Design review of the part built by this model. Coordinates are the model's own, in mm. A direction names the side the tool comes from. Round coordinates to 2 decimals unless told otherwise and drop trailing zeros. Loops run counter-clockwise (first coordinate to the right, second up) from the corner with the lowest first, then second, coordinate; pieces in that order, holes last. Notation, with made-up numbers: (68.5, 68) - (89.5, 68) arc R15 ccw to (89.5, 80) - close; hole circle Ø5 at (0.5, 21). An arc over 180 degrees is marked (long way). Return JSON: item names as keys, results as strings. Group by question number.
(1) We need section A-A, the plane x = 30. Write out the cut boundary in (y, z), and give its area (3 significant figures).
(2) The part is to be moulded in two halves that separate along Y. For faces 4 (the cylindrical face through (1, 2, 2)), 5 (the flat face through (44, 48, 4)), 6 (the flat face through (0, 65, 3)), say which applies: pulls with the +Y half, pulls with the -Y half, needs draft (parallel to the pull), parting line crosses it, or undercut.
(3) We need section B-B, the plane z = 41.5. Give the number of separate pieces and of enclosed holes in the cut face, and give its area (4 significant figures).
(4) For faces 1 (the flat face through (24, 24, 51)), 2 (the flat face through (1.5, 92, 25)), 3 (the flat face through (3, 92, 25)), list the 3-axis set-ups (+Z, -Z, +X, -X, +Y, -Y) from which the entire face can be reached by the end or side of a thin tool; tool diameter is ignored.
(5) Wall thickness on L1, parallel to X at y = 96.65, z = 25; L2, parallel to X at y = 23, z = 23.5; L3, parallel to Z at x = 60, y = 95.5: over which ranges is each line inside the solid? List them lowest first. Write a range as [from, to].
(6) We need section C-C, the plane x = 64. Write out the cut boundary in (y, z), and give its area (3 significant figures).
(7) Clearance check with flat-ended pins moving along their axes: pin 1 (3 mm diameter, centred on x = 2, z = 30, fed in from -Y); pin 2 (1.5 mm diameter, centred on x = 16.5, z = 37.5, fed in from -Y); pin 3 (2.5 mm diameter, centred on y = 92, z = 29, fed in from +X). State where each tip first meets the part, or that it passes through.
from build123d import *

# Parameters (mm, degrees)
PAD_DEPTH         = 4
SKETCH002_W       = 90
SKETCH002_H       = 4
PAD001_DEPTH      = 54
SKETCH001_W       = 5
SKETCH001_H       = 4
PAD002_DEPTH      = 51
SKETCH005_R       = 2
POCKET_DEPTH      = 84.001
POCKET_DEPTH_BACK = -14.001
SKETCH004_W       = 70
SKETCH004_H       = 1.5
PAD003_DEPTH      = 10
SKETCH003_W       = 1.5
SKETCH003_H       = 3
SKETCH003_W_2     = 2.5
SKETCH003_H_2     = 0.9
PAD004_DEPTH      = 46.5


with BuildPart() as part:
    # Sketch → Pad (new body)
    with BuildSketch(Plane.XY):
        with BuildLine():
            Line((0, 94), (0, 5))
            ThreePointArc((0, 5), (1.464466, 1.464466), (5, 0))
            Line((5, 0), (85, 0))
            ThreePointArc((85, 0), (88.535534, 1.464466), (90, 5))
            Line((90, 5), (90, 94))
            Line((90, 94), (0, 94))
        make_face()
    extrude(amount=PAD_DEPTH)

    # Sketch002 → Pad001 (join)
    with BuildSketch(Plane.XY):
        with Locations((45, 96)):
            Rectangle(SKETCH002_W, SKETCH002_H)
    extrude(amount=PAD001_DEPTH)

    # Sketch001 → Pad002 (join)
    with BuildSketch(Plane.XY):
        with Locations((17.5, 92)):
            Rectangle(SKETCH001_W, SKETCH001_H)
        with Locations((17.5, 24)):
            Rectangle(SKETCH001_W, SKETCH001_H)
        with Locations((23.7, 92)):
            Rectangle(SKETCH001_W, SKETCH001_H)
        with Locations((23.7, 24)):
            Rectangle(SKETCH001_W, SKETCH001_H)
    extrude(amount=PAD002_DEPTH)

    # Sketch005 → Pocket (cut, two sides)
    with BuildSketch(Plane(origin=(0, 84, 0), x_dir=(-1, 0, 0), z_dir=(0, 1, 0))) as pocket_sk:
        with Locations((-30, 25)):
            Circle(SKETCH005_R)
        with Locations((-60, 25)):
            Circle(SKETCH005_R)
    extrude(amount=-POCKET_DEPTH, mode=Mode.SUBTRACT)
    extrude(pocket_sk.sketch, amount=-POCKET_DEPTH_BACK, mode=Mode.SUBTRACT)

    # Sketch004 → Pad003 (join)
    with BuildSketch(Plane.XY):
        with Locations((45, 1.75)):
            Rectangle(SKETCH004_W, SKETCH004_H)
    extrude(amount=PAD003_DEPTH)

    # Sketch003 → Pad004 (join)
    with BuildSketch(Plane.XY):
        with Locations((2.25, 92.5)):
            Rectangle(SKETCH003_W, SKETCH003_H)
        with Locations((2.25, 90.55)):
            Rectangle(SKETCH003_W_2, SKETCH003_H_2)
        with Locations((87.75, 92.5)):
            Rectangle(SKETCH003_W, SKETCH003_H)
        with Locations((87.75, 90.55)):
            Rectangle(SKETCH003_W_2, SKETCH003_H_2)
    extrude(amount=PAD004_DEPTH)


solid = part.part
Solutions:
{
 "1": {"outline": "(0, 0) - (98, 0) - (98, 23) - (94, 23) - (94, 4) - (2.5, 4) - (2.5, 10) - (1, 10) - (1, 4) - (0, 4) - close; (94, 27) - (98, 27) - (98, 54) - (94, 54) - close", "area": "585 mm^2"},
 "2": {"face 4": "pulls with the -Y half", "face 5": "undercut", "face 6": "needs draft"},
 "3": {"separate pieces": "3", "enclosed holes": "0", "area": "453.5 mm^2"},
 "4": {"face 1": "+Z, +X, -X, -Y", "face 2": "+Z, -X", "face 3": "+Z"},
 "5": {"L1": "[0, 28], [32, 58], [62, 90]", "L2": "[15, 20], [21.2, 26.2]", "L3": "[0, 23], [27, 54]"},
 "6": {"outline": "(0, 0) - (98, 0) - (98, 54) - (94, 54) - (94, 4) - (2.5, 4) - (2.5, 10) - (1, 10) - (1, 4) - (0, 4) - close", "area": "601 mm^2"},
 "7": {"pin 1": "y = 90.1", "pin 2": "y = 22", "pin 3": "x = 89"}
}
